For this review, take the finished solid that the model builds, in its own axes (mm). A direction names the side the tool comes from. Give positions to 0.01 mm unless a question says otherwise; leave off trailing zeros. Loops run counter-clockwise (first coordinate to the right, second up) from the corner with the lowest first, then second, coordinate; pieces in that order, holes last. Notation, with made-up numbers: (-10, 57.25) -> (34, 57.25) arc R23 cw to (34, 65.25) -> close; hole circle Ø1 at (48, -20). An arc over 180 degrees is marked (long way). Answer as CSV lines item,"result". Start each with the question number.
Item 1: Add section A-A on z = 3.5. State the section outline as (x, y) points, plus the area to 3 significant figures.
Item 2: Add section C-C on y = 15. State the section outline as (x, z) points.
Item 3: Clearance check with a flat-ended pin moving along its axis: P1, Ø1.5, axis at x = 14.5, z = 4.5, coming from the -Y side. State where the tip first meets the part, or that it passes through.
Item 4: For L1, parallel to Y at x = 15.5, z = 3.5; L2, parallel to X at y = 25, z = 4.25; L3, parallel to X at y = 13, z = 5.25, list the stretches that pass through material, from the lowest coordinate up. Write a range as from..to.
Item 5: Machinability: for faces 1 (the face through (-16, 36.111, 4)), 2 (the face through (15, 36.111, 4)), 3 (the face through (-19.43, 75.51, 3.94)), which of the approach directions +Z, -Z, +X, -X, +Y, -Y give a long, thin tool a straight path to every point of the face, cutting with its end or side? Answer none if there is none.
Item 6: Add section B-B on x = 17. State the section outline as (y, z) points.
Autodesk Inventor part; units mm, degrees
ref_plane "YZ Plane" through (0, 0, 0) normal (1, 0, 0) x (0, 1, 0)
ref_plane "XZ Plane" through (0, 0, 0) normal (0, 1, 0) x (-1, 0, 0)
ref_plane "XY Plane" through (0, 0, 0) normal (0, 0, 1) x (1, 0, 0)
sketch "Sketch1" plane through (0, 0, 0) normal (0, 0, 1) x (1, 0, 0)
  line L0 (0, 0) -> (0, 17.1478) construction
  line L1 (-10.0548, 0.1113) -> (10.0548, 0.1113)
  line L2 (12.054, 2.0558) -> (13, 36.1113)
  line L3 (13, 36.1113) -> (18, 36.1113)
  line L4 (20, 38.1113) -> (20, 74.1113)
  line L5 (18, 76.1113) -> (-18, 76.1113)
  line L6 (-20, 74.1113) -> (-20, 38.1113)
  line L7 (-18, 36.1113) -> (-13, 36.1113)
  line L8 (-13, 36.1113) -> (-12.054, 2.0558)
  arc A0 (-18, 76.1113) -> (-20, 74.1113) centre (-18, 74.1113) ccw
  arc A1 (20, 74.1113) -> (18, 76.1113) centre (18, 74.1113) ccw
  arc A2 (-20, 38.1113) -> (-18, 36.1113) centre (-18, 38.1113) ccw
  arc A3 (18, 36.1113) -> (20, 38.1113) centre (18, 38.1113) ccw
  arc A4 (-12.054, 2.0558) -> (-10.0548, 0.1113) centre (-10.0548, 2.1113) ccw
  arc A5 (10.0548, 0.1113) -> (12.054, 2.0558) centre (10.0548, 2.1113) ccw
  point P0 (-12, 0.1113)
  point P1 (12, 0.1113)
  point P2 (20, 36.1113)
  point P3 (20, 76.1113)
  point P4 (-20, 76.1113)
  dimension "d0" = 24
  dimension "d1" = 26
  dimension "d2" = 40
  dimension "d3" = 36
  dimension "d4" = 40
  dimension "d5" = 2
extrude "Plate1" add sketch "Sketch1" along normal blind 8
equation "\"d6\" = Thickness"
equation "\"BendRadius\" = Thickness"
equation "\"BendReliefWidth\" = Thickness"
equation "\"BendReliefDepth\" = 0.5 * Thickness"
equation "\"CornerReliefSize\" = 4 * Thickness"
equation "\"MinimumRemnant\" = 2 * Thickness"
equation "\"TransitionRadius\" = BendRadius"
equation "\"JacobiRadiusSize\" = BendRadius"
equation "\"GapSize\" = Thickness"
properties part number "hage" material "S235JR"
Computed values:
1,outline,"(-20, 38.11) arc R2 ccw to (-18, 36.11) -> (-13, 36.11) -> (-12.05, 2.06) arc R2 ccw to (-10.05, 0.11) -> (10.05, 0.11) arc R2 ccw to (12.05, 2.06) -> (13, 36.11) -> (18, 36.11) arc R2 ccw to (20, 38.11) -> (20, 74.11) arc R2 ccw to (18, 76.11) -> (-18, 76.11) arc R2 ccw to (-20, 74.11) -> close"
1,area,"2,490 mm²"
2,outline,"(-12.41, 0) -> (12.41, 0) -> (12.41, 8) -> (-12.41, 8) -> close"
3,P1,"y = 36.11"
4,L1,"36.11..76.11"
4,L2,"-12.69..12.69"
4,L3,"-12.36..12.36"
5,face 1,"+Z, -Z, -X, -Y"
5,face 2,"+Z, -Z, +X, -Y"
5,face 3,"+Z, -Z, -X, +Y"
6,outline,"(36.11, 0) -> (76.11, 0) -> (76.11, 8) -> (36.11, 8) -> close"
